```python
from build123d import *

# Parameters (mm, degrees)
SCHIZZO1_W                           = 47
SCHIZZO1_H                           = 45
ESTRUSIONE_ESTRUSIONE1_DEPTH         = 16
SCHIZZO3_W                           = 5
SCHIZZO3_H                           = 9
SCHIZZO3_W_2                         = 23
TAGLIO_ESTRUSIONE1_DEPTH             = 54.228281956
TAGLIO_ESTRUSIONE2_REACH             = 52.262
SCHIZZO4_W                           = 9
SCHIZZO4_H                           = 44
TAGLIO_ESTRUSIONE3_DEPTH             = 1
FORO_PER_VITE_M3_1_D                 = 2
FORO_PER_VITE_M3_1_DEPTH             = 4
SVUOTA1_START                        = 1
SVUOTA1_DEPTH                        = 5
SCHIZZO11_W                          = 15
SCHIZZO11_H                          = 26
TAGLIO_ESTRUSIONE4_DEPTH             = 36.825968235
TAGLIO_ESTRUSIONE5_REACH             = 55.228
SCHIZZO12_W                          = 36
SCHIZZO12_H                          = 4
TAGLIO_ESTRUSIONE5_DIRECTION_2_DEPTH = 54.228281956
ESTRUSIONE_ESTRUSIONE2_DEPTH         = 6
SCHIZZO14_W                          = 1
SCHIZZO14_H                          = 2.5
TAGLIO_ESTRUSIONE6_DEPTH             = 15.26
TAGLIO_ESTRUSIONE7_REACH             = 51.482
SMUSSO1_SIZE                         = 0.5
SCHIZZO16_W                          = 4
SCHIZZO16_H                          = 1
SCHIZZO16_W_2                        = 2
SCHIZZO16_W_3                        = 20
SCHIZZO16_H_2                        = 0.8
SCHIZZO16_W_4                        = 5
SCHIZZO16_W_5                        = 13
SCHIZZO16_W_6                        = 6
SCHIZZO16_W_7                        = 1.5
ESTRUSIONE_ESTRUSIONE3_DEPTH         = 5
TAGLIO_ESTRUSIONE8_REACH             = 53.1
SCHIZZO17_W                          = 4
SCHIZZO17_H                          = 7
SCHIZZO18_W                          = 29
SCHIZZO18_H                          = 4
TAGLIO_ESTRUSIONE9_DEPTH             = 11.896238686
TAGLIO_ESTRUSIONE10_REACH            = 44.195
SCHIZZO19_W                          = 1
SCHIZZO19_H                          = 4
SCHIZZO20_R                          = 1.5
SCHIZZO20_W                          = 1
SCHIZZO20_H                          = 3
ESTRUSIONE_ESTRUSIONE4_DEPTH         = 15
TAGLIO_ESTRUSIONE11_START            = -7
SCHIZZO21_R                          = 1.5
SCHIZZO21_R_2                        = 1.3
TAGLIO_ESTRUSIONE11_DEPTH            = 7
TAGLIO_ESTRUSIONE12_START            = -3
TAGLIO_ESTRUSIONE12_DEPTH            = 3
SCHIZZO23_W                          = 1
SCHIZZO23_H                          = 6
ESTRUSIONE_ESTRUSIONE5_DEPTH         = 13
TAGLIO_ESTRUSIONE14_REACH            = 55.228


# Read off the part's stored shape, not the designer's step: Svuota1
with BuildPart() as part:
    # Schizzo1 → Estrusione-Estrusione1 (new body)
    with BuildSketch(Plane.XY):
        Rectangle(SCHIZZO1_W, SCHIZZO1_H)
    extrude(amount=ESTRUSIONE_ESTRUSIONE1_DEPTH)

    # Schizzo3 → Taglio-Estrusione1 (cut, through all)
    with BuildSketch(Plane.XZ.offset(22.5)):
        with Locations((-21, 11.5)):
            Rectangle(SCHIZZO3_W, SCHIZZO3_H)
        with Locations((12, 11.5)):
            Rectangle(SCHIZZO3_W_2, SCHIZZO3_H)
    extrude(amount=-TAGLIO_ESTRUSIONE1_DEPTH, mode=Mode.SUBTRACT)

    # Schizzo4 → Taglio-Estrusione2 (cut, up to next)
    with BuildSketch(Plane.ZY.offset(18.5), mode=Mode.PRIVATE) as taglio_estrusione2_sk1:
        with Locations((11.5, 0.5)):
            Rectangle(SCHIZZO4_W, SCHIZZO4_H)
    taglio_estrusione2_tool1 = extrude(taglio_estrusione2_sk1.sketch, amount=-TAGLIO_ESTRUSIONE2_REACH, mode=Mode.PRIVATE) & part.part
    add(taglio_estrusione2_tool1.solids().sort_by_distance((-18.5, 0.5, 11.5))[0], mode=Mode.SUBTRACT)

    # Schizzo5 → Taglio-Estrusione3 (cut)
    with BuildSketch(Plane.XY.offset(7)):
        Polygon((-18.5, -21.5), (-18.5, -22.3), (-23.3, -22.3), (-23.3, 22.3), (22.8, 22.3), (22.8, -21.8), (0.5, -21.8), (0.5, -21.5), align=None)
    extrude(amount=-TAGLIO_ESTRUSIONE3_DEPTH, mode=Mode.SUBTRACT)

    # Foro per Vite M3-1
    with Locations(Plane.XY.offset(6)):
        with Locations((-21.49, 17.25), (-21.48, -20.49), (21.49, -20.49), (21.49, 17.25)):
            Hole(FORO_PER_VITE_M3_1_D / 2, depth=FORO_PER_VITE_M3_1_DEPTH)

    # Svuota1 outline → Svuota1 (cut)
    with BuildSketch(Plane.XY.offset(SVUOTA1_START)):
        with BuildLine():
            ThreePointArc((-22.5, -18.769651198), (-20.069895601, -19.071689179), (-19.753761314, -21.5))
            Line((-19.753761314, -21.5), (19.763761314, -21.5))
            ThreePointArc((19.763761314, -21.5), (20.075786438, -19.075786438), (22.5, -18.763761314))
            Line((22.5, -18.763761314), (22.5, 15.523761314))
            ThreePointArc((22.5, 15.523761314), (19.49, 17.25), (22.5, 18.976238686))
            Line((22.5, 18.976238686), (22.5, 21.5))
            Line((22.5, 21.5), (-22.5, 21.5))
            Line((-22.5, 21.5), (-22.5, 18.976238686))
            ThreePointArc((-22.5, 18.976238686), (-19.49, 17.25), (-22.5, 15.523761314))
            Line((-22.5, 15.523761314), (-22.5, -18.769651198))
        make_face()
    extrude(amount=SVUOTA1_DEPTH, mode=Mode.SUBTRACT)

    # Schizzo11 → Taglio-Estrusione4 (cut, through all)
    with BuildSketch(Plane.XY.offset(1)):
        with Locations((9.76, -5)):
            Rectangle(SCHIZZO11_W, SCHIZZO11_H)
    extrude(amount=-TAGLIO_ESTRUSIONE4_DEPTH, mode=Mode.SUBTRACT)

    # Taglio-Estrusione5: up to this face of the body (flat: up to its plane)
    taglio_estrusione5_end = Plane(part.part.faces().sort_by_distance((0, 21.5, 3.5))[0])
    # Schizzo12 → Taglio-Estrusione5 (cut, up to the picked face)
    with BuildSketch(Plane(origin=(0, 22.5, 0), x_dir=(1, 0, 0), z_dir=(0, 1, 0)), mode=Mode.PRIVATE) as taglio_estrusione5_sk1:
        with Locations((0.5, -5)):
            Rectangle(SCHIZZO12_W, SCHIZZO12_H)
    taglio_estrusione5_tool1 = split(extrude(taglio_estrusione5_sk1.sketch, amount=-TAGLIO_ESTRUSIONE5_REACH, mode=Mode.PRIVATE), bisect_by=taglio_estrusione5_end, keep=Keep.BOTH, mode=Mode.PRIVATE)
    add(taglio_estrusione5_tool1.solids().sort_by(Axis((0.5, 22.5, 5), (0, -1, 0)))[0], mode=Mode.SUBTRACT)

    # Schizzo12 → Taglio-Estrusione5 direction 2 (cut)
    with BuildSketch(Plane(origin=(0, 22.5, 0), x_dir=(1, 0, 0), z_dir=(0, 1, 0))):
        with Locations((0.5, -5)):
            Rectangle(SCHIZZO12_W, SCHIZZO12_H)
    extrude(amount=TAGLIO_ESTRUSIONE5_DIRECTION_2_DEPTH, mode=Mode.SUBTRACT)

    # Schizzo13 → Estrusione-Estrusione2 (add)
    with BuildSketch(Plane.XY.offset(1)):
        Polygon((17.5, -21.5), (17.5, -18), (2.24, -18), (2.24, -21.5), (3.24, -21.5), (3.24, -19), (17, -19), (17, -21.5), align=None)
    extrude(amount=ESTRUSIONE_ESTRUSIONE2_DEPTH)

    # Schizzo14 → Taglio-Estrusione6 (cut)
    with BuildSketch(Plane.ZY.offset(-2.24)):
        with Locations((6.5, -20.25)):
            Rectangle(SCHIZZO14_W, SCHIZZO14_H)
    extrude(amount=-TAGLIO_ESTRUSIONE6_DEPTH, mode=Mode.SUBTRACT)

    # Schizzo15 → Taglio-Estrusione7 (cut, up to next)
    with BuildSketch(Plane(origin=(0, -18, 0), x_dir=(1, 0, 0), z_dir=(0, 1, 0)), mode=Mode.PRIVATE) as taglio_estrusione7_sk1:
        with BuildLine():
            Line((7.87, -3), (11.87, -3))
            ThreePointArc((11.87, -3), (13.620947528, -4.7133645), (14.5, -7))
            Line((14.5, -7), (5.24, -7))
            ThreePointArc((5.24, -7), (6.119052472, -4.7133645), (7.87, -3))
        make_face()
    taglio_estrusione7_tool1 = extrude(taglio_estrusione7_sk1.sketch, amount=-TAGLIO_ESTRUSIONE7_REACH, mode=Mode.PRIVATE) & part.part
    add(taglio_estrusione7_tool1.solids().sort_by_distance((9.87, -18, 5.221754))[0], mode=Mode.SUBTRACT)

    # Smusso1
    smusso1_edges = [part.edges().sort_by_distance(p)[0] for p in [
        (2.26, -5, 1),
        (17.26, -5, 1),
    ]]
    chamfer(smusso1_edges, length=SMUSSO1_SIZE)

    # Schizzo16 → Estrusione-Estrusione3 (add)
    with BuildSketch(Plane.XY.offset(1)):
        Polygon((22.5, -9.5), (22.5, -10.5), (19.5, -10.5), (19.5, -1.5), (22.5, -1.5), (22.5, -2.5), (20.5, -2.5), (20.5, -9.5), align=None)
        with Locations((20.5, 10.48)):
            Rectangle(SCHIZZO16_W, SCHIZZO16_H)
        with Locations((21.5, 8.38)):
            Rectangle(SCHIZZO16_W_2, SCHIZZO16_H)
        with Locations((-12.5, 8.28)):
            Rectangle(SCHIZZO16_W_3, SCHIZZO16_H_2)
        with Locations((-20.5, 10.38)):
            Rectangle(SCHIZZO16_W, SCHIZZO16_H_2)
        with Locations((-20, 19.376238686)):
            Rectangle(SCHIZZO16_W_4, SCHIZZO16_H_2)
        with Locations((20, 19.376238686)):
            Rectangle(SCHIZZO16_W_4, SCHIZZO16_H_2)
        with Locations((5, 19.376238686)):
            Rectangle(SCHIZZO16_W_5, SCHIZZO16_H_2)
        with Locations((8.5, 10.38)):
            Rectangle(SCHIZZO16_W_6, SCHIZZO16_H_2)
        with Locations((-9, 10.38)):
            Rectangle(SCHIZZO16_W_4, SCHIZZO16_H_2)
        with Locations((21.75, 5)):
            Rectangle(SCHIZZO16_W_7, SCHIZZO16_H)
    extrude(amount=ESTRUSIONE_ESTRUSIONE3_DEPTH)

    # Schizzo17 → Taglio-Estrusione8 (cut, up to next)
    with BuildSketch(Plane.ZY.offset(-19.5), mode=Mode.PRIVATE) as taglio_estrusione8_sk1:
        with Locations((4, -6)):
            Rectangle(SCHIZZO17_W, SCHIZZO17_H)
    taglio_estrusione8_tool1 = extrude(taglio_estrusione8_sk1.sketch, amount=-TAGLIO_ESTRUSIONE8_REACH, mode=Mode.PRIVATE) & part.part
    add(taglio_estrusione8_tool1.solids().sort_by_distance((19.5, -6, 4))[0], mode=Mode.SUBTRACT)

    # Schizzo18 → Taglio-Estrusione9 (cut)
    with BuildSketch(Plane(origin=(0, 19.776238686, 0), x_dir=(1, 0, 0), z_dir=(0, 1, 0))):
        with Locations((-3, -4)):
            Rectangle(SCHIZZO18_W, SCHIZZO18_H)
    extrude(amount=-TAGLIO_ESTRUSIONE9_DEPTH, mode=Mode.SUBTRACT)

    # Schizzo19 → Taglio-Estrusione10 (cut, up to next)
    with BuildSketch(Plane(origin=(0, 8.68, 0), x_dir=(1, 0, 0), z_dir=(0, 1, 0)), mode=Mode.PRIVATE) as taglio_estrusione10_sk1:
        with Locations((-18, -4)):
            Rectangle(SCHIZZO19_W, SCHIZZO19_H)
    taglio_estrusione10_tool1 = extrude(taglio_estrusione10_sk1.sketch, amount=-TAGLIO_ESTRUSIONE10_REACH, mode=Mode.PRIVATE) & part.part
    add(taglio_estrusione10_tool1.solids().sort_by_distance((-18, 8.68, 4))[0], mode=Mode.SUBTRACT)

    # Schizzo20 → Estrusione-Estrusione4 (add)
    with BuildSketch(Plane.XY.offset(1)):
        with Locations(Location((-19.5, 2.88, 0), (0, 0, 180))):
            Circle(SCHIZZO20_R)
        with Locations((20.5, 5)):
            Rectangle(SCHIZZO20_W, SCHIZZO20_H)
    extrude(amount=ESTRUSIONE_ESTRUSIONE4_DEPTH)

    # Schizzo21 → Taglio-Estrusione11 (cut)
    with BuildSketch(Plane.XY.offset(16).offset(TAGLIO_ESTRUSIONE11_START)):
        with Locations(Location((-19.5, 2.88, 0), (0, 0, 180))):
            Circle(SCHIZZO21_R)
        with Locations((-19.5, 2.88)):
            Circle(SCHIZZO21_R_2, mode=Mode.SUBTRACT)
    extrude(amount=TAGLIO_ESTRUSIONE11_DEPTH, mode=Mode.SUBTRACT)

    # Schizzo22 → Taglio-Estrusione12 (cut)
    with BuildSketch(Plane.XY.offset(16).offset(TAGLIO_ESTRUSIONE12_START)):
        with BuildLine():
            Line((-20.8, 2.88), (-18.2, 2.88))
            ThreePointArc((-18.2, 2.88), (-19.5, 1.58), (-20.8, 2.88))
        make_face()
    extrude(amount=TAGLIO_ESTRUSIONE12_DEPTH, mode=Mode.SUBTRACT)

    # Schizzo23 → Estrusione-Estrusione5 (add)
    with BuildSketch(Plane.XY.offset(1)):
        with Locations((-20.5, -7.5)):
            Rectangle(SCHIZZO23_W, SCHIZZO23_H)
    extrude(amount=ESTRUSIONE_ESTRUSIONE5_DEPTH)

    # Schizzo25 → Taglio-Estrusione14 (cut, up to next)
    with BuildSketch(Plane(origin=(0, 22.5, 0), x_dir=(1, 0, 0), z_dir=(0, 1, 0)), mode=Mode.PRIVATE) as taglio_estrusione14_sk1:
        with BuildLine():
            Line((14.110810194, -3), (10.011633802, -3))
            ThreePointArc((10.011633802, -3), (10.15430246, -2.745992416), (10.414334326, -2.614624125))
            ThreePointArc((10.414334326, -2.614624125), (12.289339232, -2.550566702), (14.110810194, -3))
        make_face()
    taglio_estrusione14_tool1 = extrude(taglio_estrusione14_sk1.sketch, amount=-TAGLIO_ESTRUSIONE14_REACH, mode=Mode.PRIVATE) & part.part
    add(taglio_estrusione14_tool1.solids().sort_by_distance((11.816989, 22.5, 2.796311))[0], mode=Mode.SUBTRACT)


solid = part.part
```
Geometry: final body of the model. Coordinates: model frame, mm. Coordinates: 2 decimals unless noted, no trailing zeros. Order: outer loops, then holes, each group sorted by start corner. A loop starts at its lowest first (then second) coordinate and runs counter-clockwise, first axis right, second up. Notation, with made-up numbers: M 32,-4.5 L 40,-4.5 A27 ccw 40,33.5 Z; hole C 48.25,-4 d9. An arc over 180 degrees is marked long. Answer in a Markdown table with one row per item. Add a question column.
Q1. Mould query, pull axis Y, two halves, no side actions, for faces 1 (the flat face through (2.24, -20, 4)), 2 (the cylindrical face through (20.05, -19.1, 3.46)), 3 (the flat face through (0, 22.5, 2)). Classes: released by +Y, released by -Y, zero draft, split by the parting line, or undercut.
Q2. Section query D-D on y = -5.5. Return the cut outline in (x, z), and give its area (4 significant figures).
Q3. Section query C-C on x = -4. Return the cut outline in (y, z), and give its area (3 significant figures).
Q4. Section query B-B on y = 0. Return the cut outline in (x, z), and give its area (4 significant figures).
Q5. Line query: L1, parallel to Y at x = 6.5, z = 1.5; L2, parallel to Y at x = 14.5, z = 2.5; L3, parallel to X at y = 3, z = 1.5. Output: solid intervals per line, ascending.
Q6. Contact query for flat-ended pins moving along their axis: P1, Ø1.5, axis at x = -6, z = 8.5, coming from the +Y side; P2, Ø2, axis at x = 22, y = 17, coming from the +Z side; P3, Ø1.4, axis at x = -19, y = 2, coming from the +Z side; P4, Ø5, axis at y = 16, z = 10, coming from the +X side. Output: stop coordinate, or through.
Q7. Section query A-A on z = 10.5. Return the cut outline in (x, y).
Completed:
| question | item | result |
|---|---|---|
| 1 | face 1 | undercut |
| 1 | face 2 | undercut |
| 1 | face 3 | released by +Y |
| 2 | outline | M -23.5,0 L 2.26,0 L 2.26,0.5 L 1.76,1 L -20,1 L -20,14 L -21,14 L -21,1 L -22.5,1 L -22.5,6 L -23.3,6 L -23.3,7 L -23.5,7 Z; M 17.26,0 L 23.5,0 L 23.5,7 L 22.8,7 L 22.8,6 L 22.5,6 L 22.5,1 L 20.5,1 L 20.5,2 L 19.5,2 L 19.5,1 L 17.76,1 L 17.26,0.5 Z |
| 2 | area | 56.65 mm2 |
| 3 | outline | M -22.5,0 L 22.5,0 L 22.5,3 L 21.5,3 L 21.5,1 L 8.68,1 L 8.68,2 L 7.88,2 L 7.88,1 L -21.5,1 L -21.5,16 L -22.5,16 Z |
| 3 | area | 62.8 mm2 |
| 4 | outline | M -23.5,0 L 2.26,0 L 2.26,0.5 L 1.76,1 L -22.5,1 L -22.5,6 L -23.3,6 L -23.3,7 L -23.5,7 Z; M 17.26,0 L 23.5,0 L 23.5,7 L 22.8,7 L 22.8,6 L 22.5,6 L 22.5,1 L 17.76,1 L 17.26,0.5 Z |
| 4 | area | 42.65 mm2 |
| 5 | L1 | y = -22.5 to -21.5, -19 to -18, 9.98 to 10.78, 18.98 to 19.78, 21.5 to 22.5 |
| 5 | L2 | y = -22.5 to -21.5, -19 to -18, 21.5 to 22.5 |
| 5 | L3 | x = -23.5 to -22.5, -21 to -18, 22.5 to 23.5 |
| 6 | P1 | stops at y = -21.5 |
| 6 | P2 | stops at z = 7 |
| 6 | P3 | stops at z = 13 |
| 6 | P4 | passes through |
| 7 | outline | M -21,-10.5 L -20,-10.5 L -20,-4.5 L -21,-4.5 Z; C -19.5,2.88 d2.6; M -18.5,-22.5 L 0.5,-22.5 L 0.5,-21.5 L -18.5,-21.5 Z; M 20,3.5 L 21,3.5 L 21,6.5 L 20,6.5 Z |
